For this review, take the finished solid that the model builds, in its own axes (mm). A direction names the side the tool comes from. Coordinates: 2 decimals unless noted, no trailing zeros. Loops run counter-clockwise (first coordinate to the right, second up) from the corner with the lowest first, then second, coordinate; pieces in that order, holes last. Notation, with made-up numbers: M -34,40.5 L 18,40.5 A4 cw 18,44.5 Z; hole C -31,19.5 d10. An arc over 180 degrees is marked long. Answer as a JSON object with one key per item and string values. Group by question number.
Item 1: Add section C-C (y = 22.5). State the section outline as (x, z) points, then the cut area to 3 significant figures.
Item 2: Wall thickness on L1, parallel to X at y = -43, z = 1.2; L2, parallel to Y at x = 57, z = 2; L3, parallel to Y at x = 163, z = 1.2: over which ranges is each line inside the solid? List them lowest first. Write a range as from..to.
Item 3: Add section B-B (z = 0.65). Count the separate pieces of the cut face and the enclosed holes in it, then the cut area to 3 significant figures.
Item 4: Insertion check: pin 1 (1.5 mm diameter, centred on x = 181, z = 2, fed in from -Y); pin 2 (1.5 mm diameter, centred on y = -87, z = 2.5, fed in from -X); pin 3 (0.9 mm diameter, centred on y = -52.5, z = 1, fed in from -X). Each pin has a flat end and moves straight along its axis. Give the tip position at first contact, or say it passes through.
Item 5: Add section A-A (y = -93.5). State the section outline as (x, z) points.
Item 6: Tool access review of faces 5 (the face through (104, -58, 0)), 6 (the face through (18.725, -61.93, 1.521)): name each direction out of +Z, -Z, +X, -X, +Y, -Y from which nothing blocks a thin tool from reaching the whole face with its end or side.
Item 7: Mouldability with a two-part tool opening along Y and no side actions: class faces 1 (the face through (2.7, -42.3, 1.5)), 2 (the face through (109.88, -52.08, 1.52)), 3 (the face through (27.67, -51.76, 1.52)), 4 (the face through (82.924, -119.159, 1.521)) as +Y half, -Y half, draft (parallel to the pull), parting line (faces both ways), or undercut.
from build123d import *

# Parameters (mm, degrees)
SKETCH_1_R          = 7.65
EXTRUDE_1_DEPTH     = 3
FILLET_1_R          = 10
SKETCH_3_R          = 1.65
CUT_EXTRUDE_2_DEPTH = 276.061811235
FILLET_2_R          = 40
FILLET_3_R          = 80
SKETCH_4_W          = 12
SKETCH_4_H          = 3.5
EXTRUDE_2_DEPTH     = 3
CUT_EXTRUDE_3_DEPTH = 10
FILLET_4_R          = 2
FILLET_5_R          = 8
SKETCH_6_R          = 1.65
SKETCH_6_W          = 20.2
SKETCH_6_H          = 20.2
CUT_EXTRUDE_4_DEPTH = 277.6699297


with BuildPart() as part:
    # 草图1 → 凸台-拉伸1 (new body)
    with BuildSketch(Plane.XY):
        with BuildLine():
            Line((108.946536832, -55), (24.071062677, 25.408343937))
            ThreePointArc((24.071062677, 25.408343937), (-25.408343937, 24.071062677), (-24.071062677, -25.408343937))
            Line((-24.071062677, -25.408343937), (81.053463168, -125))
            Line((81.053463168, -125), (245, -125))
            Line((245, -125), (245, -55))
            Line((245, -55), (108.946536832, -55))
        make_face()
        Circle(SKETCH_1_R, mode=Mode.SUBTRACT)
    extrude(amount=EXTRUDE_1_DEPTH)

    # 圆角1
    fillet_1_edges = [part.edges().sort_by_distance(p)[0] for p in [
        (245, -55, 1.5),
        (245, -125, 1.5),
    ]]
    fillet(fillet_1_edges, radius=FILLET_1_R)

    # 草图3 → 切除-拉伸2 (cut, through all)
    with BuildSketch(Plane.XY.offset(3)):
        with Locations((10.675325257, -52.127223508)):
            Circle(SKETCH_3_R)
        with Locations((52.62774878, -7.84410979)):
            Circle(SKETCH_3_R)
        with Locations((70.824604166, -24.986876604)):
            Circle(SKETCH_3_R)
        with Locations((28.872180643, -69.269990322)):
            Circle(SKETCH_3_R)
        with BuildLine():
            Line((40.259807528, 6.14576259), (49.116430272, -2.244722115))
            ThreePointArc((49.116430272, -2.244722115), (49.179473531, -4.577322712), (46.846872934, -4.640365972))
            Line((46.846872934, -4.640365972), (37.99025019, 3.750118733))
            ThreePointArc((37.99025019, 3.750118733), (37.92720693, 6.08271933), (40.259807528, 6.14576259))
        make_face()
        with BuildLine():
            Line((16.504239392, -55.280117943), (25.360862135, -63.670602647))
            ThreePointArc((25.360862135, -63.670602647), (25.423905395, -66.003203245), (23.091304797, -66.066246504))
            Line((23.091304797, -66.066246504), (14.234682054, -57.6757618))
            ThreePointArc((14.234682054, -57.6757618), (14.171638794, -55.343161202), (16.504239392, -55.280117943))
        make_face()
        Polygon((208.35, -55), (208.35, -58.5), (206.75, -58.5), (206.75, -62), (208.35, -62), (208.35, -65.4), (211.65, -65.4), (211.65, -62), (213.25, -62), (213.25, -58.5), (211.65, -58.5), (211.65, -55), align=None)
        with BuildLine():
            Line((-1.692615995, -38.137351128), (7.164006749, -46.527835833))
            ThreePointArc((7.164006749, -46.527835833), (7.227050008, -48.86043643), (4.894449411, -48.92347969))
            Line((4.894449411, -48.92347969), (-3.962173333, -40.532994985))
            ThreePointArc((-3.962173333, -40.532994985), (-4.025216592, -38.200394388), (-1.692615995, -38.137351128))
        make_face()
        with BuildLine():
            Line((58.456662914, -10.997004225), (67.313285658, -19.387488929))
            ThreePointArc((67.313285658, -19.387488929), (67.376328917, -21.720089527), (65.04372832, -21.783132786))
            Line((65.04372832, -21.783132786), (56.187105576, -13.392648081))
            ThreePointArc((56.187105576, -13.392648081), (56.124062317, -11.060047484), (58.456662914, -10.997004225))
        make_face()
        with BuildLine():
            Line((34.701094778, -72.422884757), (43.557717522, -80.813369462))
            ThreePointArc((43.557717522, -80.813369462), (43.620760781, -83.145970059), (41.288160183, -83.209013319))
            Line((41.288160183, -83.209013319), (32.43153744, -74.818528614))
            ThreePointArc((32.43153744, -74.818528614), (32.36849418, -72.485928017), (34.701094778, -72.422884757))
        make_face()
        with BuildLine():
            Line((76.6535183, -28.139771039), (85.510141044, -36.530255744))
            ThreePointArc((85.510141044, -36.530255744), (85.573184303, -38.862856341), (83.240583706, -38.9258996))
            Line((83.240583706, -38.9258996), (74.383960962, -30.535414896))
            ThreePointArc((74.383960962, -30.535414896), (74.320917703, -28.202814298), (76.6535183, -28.139771039))
        make_face()
        Polygon((208.35, -125), (211.65, -125), (211.65, -121.5), (213.25, -121.5), (213.25, -118), (211.65, -118), (211.65, -114.6), (208.35, -114.6), (208.35, -118), (206.75, -118), (206.75, -121.5), (208.35, -121.5), align=None)
    extrude(amount=-CUT_EXTRUDE_2_DEPTH, mode=Mode.SUBTRACT)

    # 圆角2
    fillet_2_edges = [part.edges().sort_by_distance(p)[0] for p in [
        (108.946536832, -55, 1.5),
    ]]
    fillet(fillet_2_edges, radius=FILLET_2_R)

    # 圆角3
    fillet_3_edges = [part.edges().sort_by_distance(p)[0] for p in [
        (81.053463168, -125, 1.5),
    ]]
    fillet(fillet_3_edges, radius=FILLET_3_R)

    # 草图4 → 凸台-拉伸2 (add)
    with BuildSketch(Plane.XY.offset(3)):
        with Locations((229, -53.25)):
            Rectangle(SKETCH_4_W, SKETCH_4_H)
        with Locations((191, -53.25)):
            Rectangle(SKETCH_4_W, SKETCH_4_H)
        with Locations((191, -126.75)):
            Rectangle(SKETCH_4_W, SKETCH_4_H)
        with Locations((229, -126.75)):
            Rectangle(SKETCH_4_W, SKETCH_4_H)
    extrude(amount=-EXTRUDE_2_DEPTH)

    # 草图5 → 切除-拉伸3 (cut)
    with BuildSketch(Plane.XY.offset(3)):
        Polygon((36.127453438, -34.086875982), (30.735876382, -2.464353083), (4.227694858, -30.445211358), align=None)
        Polygon((41.063366277, -63.036850208), (13.12952951, -39.513402443), (37.527548139, -42.298671213), align=None)
        Polygon((44.40399322, -35.031722698), (69.950424768, -37.948093861), (39.465464045, -6.066403216), align=None)
        Polygon((51.215235175, -74.980823394), (45.804087921, -43.243517929), (77.819635369, -46.898400967), align=None)
        Polygon((102.632901746, -60.038663458), (63.421774999, -76.636422834), (90.255116273, -48.312340378), align=None)
        Polygon((99.509947592, -67.875977962), (53.116905285, -87.513785309), (81.115387776, -114.038663458), align=None)
        Polygon((88.547109373, -117), (107.005723407, -70.676565087), (170.216089142, -117), align=None)
        Polygon((183.75, -117), (110.064623342, -63), (183.75, -63), align=None)
    extrude(amount=-CUT_EXTRUDE_3_DEPTH, mode=Mode.SUBTRACT)

    # 圆角4
    fillet_4_edges = [part.edges().sort_by_distance(p)[0] for p in [
        (51.215235175, -74.980823394, 1.5),
        (45.804087921, -43.243517929, 1.5),
        (77.819635369, -46.898400967, 1.5),
        (102.632901746, -60.038663458, 1.5),
        (63.421774999, -76.636422834, 1.5),
        (90.255116273, -48.312340378, 1.5),
        (69.950424768, -37.948093861, 1.5),
        (44.40399322, -35.031722698, 1.5),
        (39.465464045, -6.066403216, 1.5),
        (41.063366277, -63.036850208, 1.5),
        (13.12952951, -39.513402443, 1.5),
        (37.527548139, -42.298671213, 1.5),
        (183.75, -117, 1.5),
        (110.064623342, -63, 1.5),
        (183.75, -63, 1.5),
        (53.116905285, -87.513785309, 1.5),
        (99.509947592, -67.875977962, 1.5),
        (107.005723407, -70.676565087, 1.5),
        (170.216089142, -117, 1.5),
        (30.735876382, -2.464353083, 1.5),
        (36.127453438, -34.086875982, 1.5),
        (4.227694858, -30.445211358, 1.5),
    ]]
    fillet(fillet_4_edges, radius=FILLET_4_R)

    # 圆角5
    fillet_5_edges = [part.edges().sort_by_distance(p)[0] for p in [
        (81.115387776, -114.038663458, 1.5),
        (88.547109373, -117, 1.5),
    ]]
    fillet(fillet_5_edges, radius=FILLET_5_R)

    # 草图6 → 切除-拉伸4 (cut, through all)
    with BuildSketch(Plane.XY.offset(3)):
        with Locations((-15.1, 0)):
            Circle(SKETCH_6_R)
        with Locations((15.1, 0)):
            Circle(SKETCH_6_R)
        Rectangle(SKETCH_6_W, SKETCH_6_H)
    extrude(amount=-CUT_EXTRUDE_4_DEPTH, mode=Mode.SUBTRACT)


solid = part.part
From the geometry:
{
 "1": {"outline": "M -26.81,0 L 27.14,0 L 27.14,3 L -26.81,3 Z", "area": "162 mm²"},
 "2": {"L1": "x = -5.5..-1.36, 3.44..17.63, 37.47..96.28", "L2": "y = -102.21..-91.19, -85.87..-68.87, -44.52..-36.47, -24.4..-14.16, -10.58..-5.79", "L3": "y = -125..-117, -111.71..-101.79, -63..-55"},
 "3": {"separate pieces": "1", "enclosed holes": "21", "area": "14,200 mm²"},
 "4": {"pin 1": "stops at y = -125", "pin 2": "stops at x = 40.15", "pin 3": "stops at x = 4.05"},
 "5": {"outline": "M 47.8,0 L 59.44,0 L 59.44,3 L 47.8,3 Z; M 89.3,0 L 97.91,0 L 97.91,3 L 89.3,3 Z; M 138.15,0 L 151.68,0 L 151.68,3 L 138.15,3 Z; M 183.75,0 L 245,0 L 245,3 L 183.75,3 Z"},
 "6": {"face 5": "-Z, +X, -X, +Y, -Y", "face 6": "+Z, -Z"},
 "7": {"face 1": "undercut", "face 2": "+Y half", "face 3": "undercut", "face 4": "-Y half"}
}
